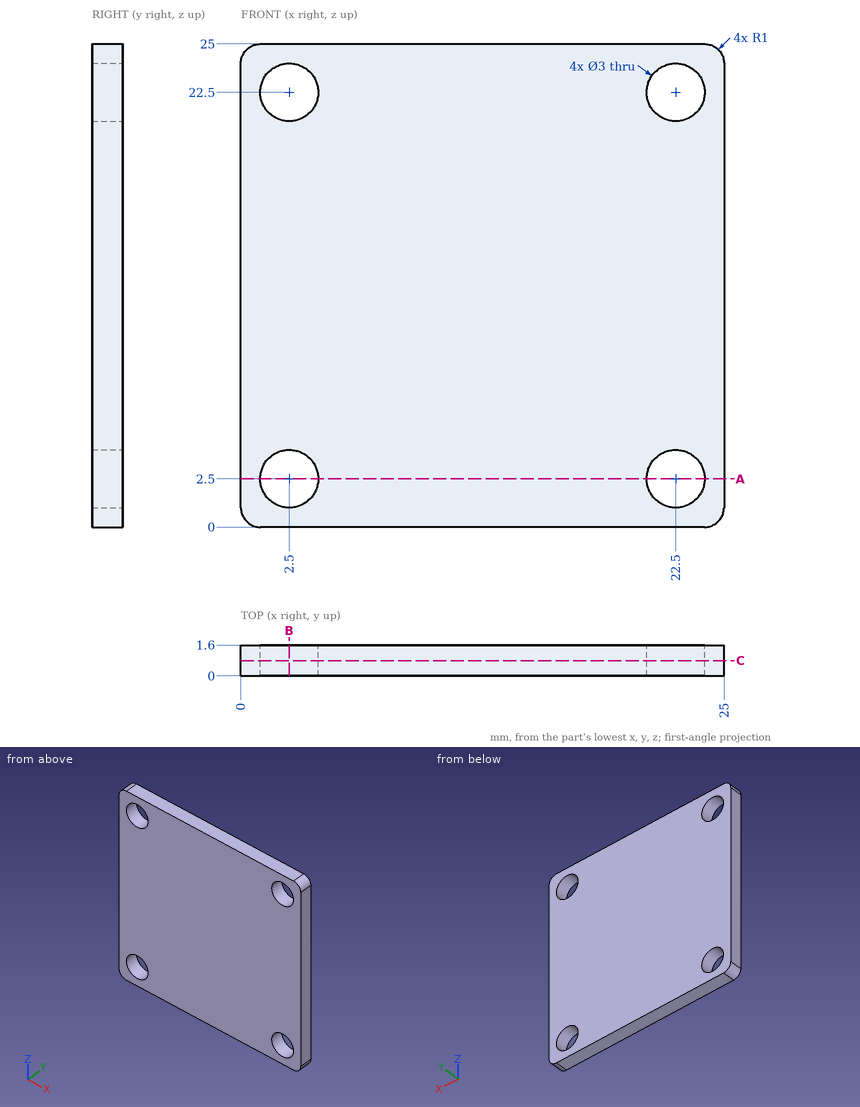
Study the drawing (mm; zero at the part's minimum x, y, z) and answer. Give positions to 0.01 mm unless a question says otherwise; leave off trailing zeros. Write each loop counter-clockwise with the first axis right and the second up, starting at its lowest first coordinate (ties: lowest second). Pieces come first, ordered by that corner, then holes. Notation, with made-up numbers: (74, -16.5) - (78, -16.5) arc R32 cw to (78, 11.5) - close; hole circle Ø10 at (-11, 32.25). An arc over 180 degrees is marked (long way). Use CSV: the item, a comma, the result in double quotes. Start each with the question number.
(1) Find section B-B (x = 2.5). Give the vertices of the cut face in (y, z), plus the area to 3 significant figures.
(2) Consider line 1 along X through (y, z) = (0.95, 2.5). Determine where the line is inside the solid, lowest interval first.
(3) Find section C-C (y = 0.8). Give the vertices of the cut face in (x, z).
(4) Find section A-A (z = 2.5). Give the vertices of the cut face in (x, y).
Findings below:
1,outline,"(0, 0) - (1.6, 0) - (1.6, 1) - (0, 1) - close; (0, 4) - (1.6, 4) - (1.6, 21) - (0, 21) - close; (0, 24) - (1.6, 24) - (1.6, 25) - (0, 25) - close"
1,area,"30.4 mm2"
2,line 1,"0 to 1, 4 to 21, 24 to 25"
3,outline,"(0, 1) arc R1 ccw to (1, 0) - (24, 0) arc R1 ccw to (25, 1) - (25, 24) arc R1 ccw to (24, 25) - (1, 25) arc R1 ccw to (0, 24) - close; hole circle Ø3 at (2.5, 2.5); hole circle Ø3 at (2.5, 22.5); hole circle Ø3 at (22.5, 2.5); hole circle Ø3 at (22.5, 22.5)"
4,outline,"(0, 0) - (1, 0) - (1, 1.6) - (0, 1.6) - close; (4, 0) - (21, 0) - (21, 1.6) - (4, 1.6) - close; (24, 0) - (25, 0) - (25, 1.6) - (24, 1.6) - close"
